The model under review builds one solid part; all positions refer to its coordinate system, in mm. A direction names the side the tool comes from. Give positions to 0.01 mm unless a question says otherwise; leave off trailing zeros. Order: outer loops, then holes, each group sorted by start corner. A loop starts at its lowest first (then second) coordinate and runs counter-clockwise, first axis right, second up.
```python
from build123d import *

# Parameters (mm, degrees)
BOX_W           = 78
BOX_H           = 108.5
BOX_DEPTH       = 74
SKETCH_W        = 72
SKETCH_H        = 50
POCKET_DEPTH    = 105.5
SKETCH001_W     = 72
SKETCH001_H     = 15
POCKET001_DEPTH = 105.5
SKETCH002_W     = 52
SKETCH002_H     = 3
POCKET002_DEPTH = 105.5
SKETCH008_W     = 75
SKETCH008_H     = 1.5
POCKET005_DEPTH = 72
SKETCH009_W     = 10
SKETCH009_H     = 3
POCKET006_DEPTH = 5
SKETCH010_W     = 10
SKETCH010_H     = 3
POCKET007_DEPTH = 5
SKETCH011_W     = 72
SKETCH011_H     = 3
POCKET008_DEPTH = 2.5
FILLET_R        = 5
SKETCH018_W     = 40
SKETCH018_H     = 3
PAD_DEPTH       = 25
SKETCH019_W     = 40
SKETCH019_H     = 3
PAD001_DEPTH    = 25
SKETCH020_W     = 5
SKETCH020_H     = 33
POCKET010_DEPTH = 3.001
SKETCH021_W     = 5
SKETCH021_H     = 33
POCKET011_DEPTH = 3.001
FILLET002_R     = 2
FILLET003_R     = 6


with BuildPart() as part:
    # Box → Box (new body)
    with BuildSketch(Plane.XY):
        with Locations((39, 54.25)):
            Rectangle(BOX_W, BOX_H)
    extrude(amount=BOX_DEPTH)

    # Sketch (on Face3 of BaseFeature) → Pocket (cut)
    with BuildSketch(Plane.XZ):
        with Locations((39, 46)):
            Rectangle(SKETCH_W, SKETCH_H)
    extrude(amount=-POCKET_DEPTH, mode=Mode.SUBTRACT)

    # Sketch001 (on Face2 of Pocket) → Pocket001 (cut)
    with BuildSketch(Plane.XZ):
        with Locations((39, 10.5)):
            Rectangle(SKETCH001_W, SKETCH001_H)
    extrude(amount=-POCKET001_DEPTH, mode=Mode.SUBTRACT)

    # Sketch002 (on Face2 of Pocket001) → Pocket002 (cut)
    with BuildSketch(Plane.XZ):
        with Locations((39, 19.5)):
            Rectangle(SKETCH002_W, SKETCH002_H)
    extrude(amount=-POCKET002_DEPTH, mode=Mode.SUBTRACT)

    # Sketch008 (on Face3 of Pocket002) → Pocket005 (cut)
    with BuildSketch(Plane.XY.offset(74)):
        with Locations((39, 1.75)):
            Rectangle(SKETCH008_W, SKETCH008_H)
    extrude(amount=-POCKET005_DEPTH, mode=Mode.SUBTRACT)

    # Sketch009 (on Face2 of Pocket005) → Pocket006 (cut)
    with BuildSketch(Plane.XZ):
        with Locations((8, 19.5)):
            Rectangle(SKETCH009_W, SKETCH009_H)
    extrude(amount=-POCKET006_DEPTH, mode=Mode.SUBTRACT)

    # Sketch010 (on Face2 of Pocket006) → Pocket007 (cut)
    with BuildSketch(Plane.XZ):
        with Locations((70, 19.5)):
            Rectangle(SKETCH010_W, SKETCH010_H)
    extrude(amount=-POCKET007_DEPTH, mode=Mode.SUBTRACT)

    # Sketch011 (on Face2 of Pocket007) → Pocket008 (cut)
    with BuildSketch(Plane.XZ):
        with Locations((39, 72.5)):
            Rectangle(SKETCH011_W, SKETCH011_H)
    extrude(amount=-POCKET008_DEPTH, mode=Mode.SUBTRACT)

    # Fillet
    fillet_edges = [part.edges().sort_by_distance(p)[0] for p in [
        (39, 108.5, 74),
        (78, 108.5, 37),
        (39, 108.5, 0),
        (0, 108.5, 37),
        (78, 54.25, 74),
        (0, 54.25, 74),
    ]]
    fillet(fillet_edges, radius=FILLET_R)

    # Sketch018 (on Face6 of Fillet) → Pad (join)
    with BuildSketch(Plane.YZ.offset(78)):
        with Locations((51.75, 1.5)):
            Rectangle(SKETCH018_W, SKETCH018_H)
    extrude(amount=PAD_DEPTH)

    # Sketch019 (on Face1 of Pad) → Pad001 (join)
    with BuildSketch(Plane(origin=(0, 0, 0), x_dir=(0, -1, 0), z_dir=(-1, 0, 0))):
        with Locations((-51.75, 1.5)):
            Rectangle(SKETCH019_W, SKETCH019_H)
    extrude(amount=PAD001_DEPTH)

    # Sketch020 (on Face32 of Pad001) → Pocket010 (cut, through all)
    with BuildSketch(Plane.XY.offset(3)):
        with Locations((96.75, 51.75)):
            Rectangle(SKETCH020_W, SKETCH020_H)
    extrude(amount=-POCKET010_DEPTH, mode=Mode.SUBTRACT)

    # Sketch021 (on Face6 of Pocket010) → Pocket011 (cut, through all)
    with BuildSketch(Plane.XY.offset(3)):
        with Locations((-18.75, 51.75)):
            Rectangle(SKETCH021_W, SKETCH021_H)
    extrude(amount=-POCKET011_DEPTH, mode=Mode.SUBTRACT)

    # Fillet002
    fillet002_edges = [part.edges().sort_by_distance(p)[0] for p in [
        (99.25, 68.25, 1.5),
        (99.25, 35.25, 1.5),
        (94.25, 35.25, 1.5),
        (94.25, 68.25, 1.5),
        (-21.25, 68.25, 1.5),
        (-16.25, 68.25, 1.5),
        (-16.25, 35.25, 1.5),
        (-21.25, 35.25, 1.5),
    ]]
    fillet(fillet002_edges, radius=FILLET002_R)

    # Fillet003
    fillet003_edges = [part.edges().sort_by_distance(p)[0] for p in [
        (103, 71.75, 1.5),
        (103, 31.75, 1.5),
        (-25, 71.75, 1.5),
        (-25, 31.75, 1.5),
    ]]
    fillet(fillet003_edges, radius=FILLET003_R)


solid = part.part
```
Item 1: Take a section at A-A (y = 60.5). Give the number of separate pieces and of enclosed holes in the cut face, and give its area (3 significant figures).
Values found:
separate pieces: 3
enclosed holes: 1
area: 1,050 mm2
Item 2: Take a section at D-D (x = 8.5). Give the boundary of the cut face in (y, z).
Values found:
outline: (0, 0) - (103.5, 0) arc R5 ccw to (108.5, 5) - (108.5, 69) arc R5 ccw to (103.5, 74) - (2.5, 74) - (2.5, 71) - (105.5, 71) - (105.5, 21) - (5, 21) - (5, 18) - (105.5, 18) - (105.5, 3) - (2.5, 3) - (2.5, 2) - (1, 2) - (1, 3) - (0, 3) - close
Item 3: Clearance check with flat-ended pins moving along their axes: pin 1 Ø3.5 at (x, z) = (-9, 1) entering from +Y; pin 2 Ø8 at (x, y) = (7.5, 55) entering from -Z; pin 3 Ø0.5 at (y, z) = (0.5, 32.5) entering from -X; pin 4 Ø1.2 at (y, z) = (2, 36.5) entering from +X. State where each tip first meets the part, or that it passes through.
Values found:
pin 1: stops at y = 71.75
pin 2: stops at z = 0
pin 3: stops at x = 0
pin 4: stops at x = 78
Item 4: Take a section at C-C (z = 15). Give the boundary of the cut face in (x, y), and give its area (3 significant figures).
Values found:
outline: (0, 0) - (3, 0) - (3, 1) - (1.5, 1) - (1.5, 2.5) - (3, 2.5) - (3, 105.5) - (75, 105.5) - (75, 2.5) - (76.5, 2.5) - (76.5, 1) - (75, 1) - (75, 0) - (78, 0) - (78, 103.5) arc R5 ccw to (73, 108.5) - (5, 108.5) arc R5 ccw to (0, 103.5) - close
area: 852 mm2
Item 5: Draft analysis for pull direction X (two halves, no side actions). For faces 1 (the flat face through (65, 55, 19)), 2 (the flat face through (103, 52, 2)), 3 (the flat face through (13, 55, 19)), 4 (the flat face through (87, 31.75, 1)), state which applies: released by +X, released by -X, zero draft, split by the parting line, or undercut.
Values found:
face 1: undercut
face 2: released by +X
face 3: undercut
face 4: zero draft
Item 6: For line 1 (Z direction, x = 70, y = 21); line 2 (X direction, y = 44, z = 63); line 3 (Z direction, x = 21, y = 54), list the stretches that pass through material, from the lowest coordinate up.
Values found:
line 1: z = 0 to 3, 18 to 21, 71 to 74
line 2: x = 0 to 3, 75 to 78
line 3: z = 0 to 3, 71 to 74
Item 7: Take a section at B-B (y = 27). Give the boundary of the cut face in (x, z), and give its area (3 significant figures).
Values found:
outline: (0, 0) - (78, 0) - (78, 69) arc R5 ccw to (73, 74) - (5, 74) arc R5 ccw to (0, 69) - close; hole (3, 3) - (75, 3) - (75, 18) - (65, 18) - (65, 21) - (75, 21) - (75, 71) - (3, 71) - (3, 21) - (13, 21) - (13, 18) - (3, 18) - close
area: 925 mm2
Item 8: For faces 5 (the flat face through (-9, 71.75, 1)), 6 (the flat face through (-9, 31.75, 1)), 7 (the flat face through (2.7, 1, 38)), 8 (the flat face through (38, 52, 0)), 9 (the flat face through (38, 53, 71)), list the 3-axis set-ups (+Z, -Z, +X, -X, +Y, -Y) from which the entire face can be reached by the end or side of a thin tool; tool diameter is ignored.
Values found:
face 5: +Z, -Z, -X, +Y
face 6: +Z, -Z, -X, -Y
face 7: +Z
face 8: -Z, +X, -X, +Y, -Y
face 9: -Y
